Check sheet for the modelled part. Datum: model origin and axes. Units: mm. A direction names the side the tool comes from. Round coordinates to 2 decimals unless told otherwise and drop trailing zeros. Write each loop counter-clockwise with the first axis right and the second up, starting at its lowest first coordinate (ties: lowest second). Pieces come first, ordered by that corner, then holes.
Item 1: Section check B-B, the plane y = 6.5. Record the cut outline in (x, z).
Item 2: Material ranges on line 1 along X through (y, z) = (1.25, 3.5); line 2 along X through (y, z) = (6.25, -0.25); line 3 along Y through (x, z) = (1, 1.5), recorded low to high.
Item 3: Release check for a two-part mould opening along X. For faces 1 (the flat face through (3, 0, 1)), 2 (the flat face through (6.288, 1, 2)), 3 (the flat face through (5, 1, -1.25)) record: pulls with the +X half, pulls with the -X half, needs draft (parallel to the pull), parting line crosses it, or undercut.
Item 4: Section check A-A, the plane z = -2. Record the cut outline in (x, y).
Item 5: Set-up check for faces 4 (the flat face through (3, 1, -1.25)), 5 (the flat face through (3, 1, 3.75)), 6 (the flat face through (-1.182, 1, 3)): record each of +Z, -Z, +X, -X, +Y, -Y from which the full face is reachable in a straight line by a thin tool's end or side.
Item 6: Depth check by flat-ended pin: pin 1 (0.7 mm diameter, centred on y = -0.5, z = -1, fed in from +X); pin 2 (0.8 mm diameter, centred on x = 0, y = 0.5, fed in from -Z); pin 3 (0.5 mm diameter, centred on y = 6, z = 2.5, fed in from -X). Enter the tip coordinate at first touch or a pass-through.
from build123d import *

# Parameters (mm, degrees)
BOSS_EXTRUDE3_DEPTH = 2.54
BOSS_EXTRUDE4_DEPTH = 2.54
LPATTERN1_COUNT     = 2
LPATTERN1_PITCH     = 2.54
BOSS_EXTRUDE5_DEPTH = 0.32
CHAMFER1_SIZE       = 0.16
CHAMFER1_SIZE2      = 0.5458
LPATTERN2_START     = 2.38
LPATTERN2_DEPTH     = 0.32
LPATTERN2_START_2   = 4.92
LPATTERN2_2_DEPTH   = 0.32
LPATTERN2_START_3   = 2.22
LPATTERN2_3_DEPTH   = 0.64
LPATTERN2_START_4   = 4.76
LPATTERN2_4_DEPTH   = 0.64
LPATTERN2_START_5   = -0.32
LPATTERN2_5_DEPTH   = 0.64
LPATTERN2_START_6   = 1
LPATTERN2_6_DEPTH   = 5
SKETCH9_W           = 6.730038924
SKETCH9_H           = 1
BOSS_EXTRUDE6_DEPTH = 2.54


with BuildPart() as part:
    # Sketch6 → Boss-Extrude3 (new body)
    with BuildSketch(Plane(origin=(0, 0, 0), x_dir=(1, 0, 0), z_dir=(0, 1, 0))):
        Polygon((-1.1825, 0.75), (-1.1825, -0.75), (-0.812519462, -1.25), (0.812519462, -1.25), (1.1825, -0.75), (1.1825, 0.75), (0.812519462, 1.25), (-0.812519462, 1.25), align=None)
    extrude(amount=BOSS_EXTRUDE3_DEPTH)

    # Sketch7 → Boss-Extrude4 (add)
    with BuildSketch(Plane(origin=(0, 0, 0), x_dir=(1, 0, 0), z_dir=(0, 1, 0))):
        Polygon((1.1825, 0.75), (1.1825, -0.75), (1.3825, -0.75), (1.752480538, -1.25), (3.377519462, -1.25), (3.7475, -0.75), (3.7475, 0.75), (3.377519462, 1.25), (1.752480538, 1.25), (1.3825, 0.75), align=None)
    boss_extrude4 = extrude(amount=BOSS_EXTRUDE4_DEPTH)

    # LPattern1: Boss-Extrude4 ×2
    with Locations(*[(i * LPATTERN1_PITCH, 0, 0) for i in range(1, LPATTERN1_COUNT)]):
        add(boss_extrude4)

    # Sketch8 → Boss-Extrude5 (add, symmetric)
    with BuildSketch(Plane(origin=(0, 0, 0), x_dir=(0, 0, -1), z_dir=(1, 0, 0))):
        with BuildLine():
            Line((0.32, 0), (0.32, 8))
            Line((0.32, 8), (-0.32, 8))
            Line((-0.32, 8), (-0.32, 0))
            ThreePointArc((-0.32, 0), (-0.13254834, -0.45254834), (0.32, -0.64))
            Line((0.32, -0.64), (2.5, -0.64))
            Line((2.5, -0.64), (2.5, 0))
            Line((2.5, 0), (0.32, 0))
        make_face()
    extrude(amount=BOSS_EXTRUDE5_DEPTH, both=True)

    # Chamfer1
    chamfer1_edges = [part.edges().sort_by_distance(p)[0] for p in [
        (-0.32, 8, 0),
        (0, 8, -0.32),
        (0, 8, 0.32),
        (0.32, 8, 0),
    ]]
    chamfer1_side = [part.faces().sort_by_distance(p)[0] for p in [
        (0, 8, 0),
    ]]
    chamfer(chamfer1_edges, length=CHAMFER1_SIZE, length2=CHAMFER1_SIZE2, reference=chamfer1_side[0])

    # LPattern2: read off the stored shape, not the designer's step
    # LPattern2 outline → LPattern2 (add)
    with BuildSketch(Plane.YZ.offset(LPATTERN2_START)):
        with BuildLine():
            Line((-0.64, -0.32), (-0.64, -2.5))
            Line((-0.64, -2.5), (0, -2.5))
            Line((0, -2.5), (0, 0.32))
            ThreePointArc((0, 0.32), (-0.45254834, 0.13254834), (-0.64, -0.32))
        make_face()
        Polygon((2.54, -0.32), (7.4542, -0.32), (8, -0.16), (8, 0.16), (7.4542, 0.32), (2.54, 0.32), align=None)
    extrude(amount=LPATTERN2_DEPTH)

    # LPattern2 2 outline → LPattern2 2 (add)
    with BuildSketch(Plane.YZ.offset(LPATTERN2_START_2)):
        with BuildLine():
            Line((-0.64, -0.32), (-0.64, -2.5))
            Line((-0.64, -2.5), (0, -2.5))
            Line((0, -2.5), (0, 0.32))
            ThreePointArc((0, 0.32), (-0.45254834, 0.13254834), (-0.64, -0.32))
        make_face()
        Polygon((2.54, -0.32), (7.4542, -0.32), (8, -0.16), (8, 0.16), (7.4542, 0.32), (2.54, 0.32), align=None)
    extrude(amount=LPATTERN2_2_DEPTH)

    # LPattern2 3 outline → LPattern2 3 (add)
    with BuildSketch(Plane.YZ.offset(LPATTERN2_START_3)):
        with BuildLine():
            Line((-0.64, -0.32), (-0.64, -2.5))
            Line((-0.64, -2.5), (0, -2.5))
            Line((0, -2.5), (0, 0.32))
            ThreePointArc((0, 0.32), (-0.45254834, 0.13254834), (-0.64, -0.32))
        make_face()
    extrude(amount=LPATTERN2_3_DEPTH)

    # LPattern2 4 outline → LPattern2 4 (add)
    with BuildSketch(Plane.YZ.offset(LPATTERN2_START_4)):
        with BuildLine():
            Line((-0.64, -0.32), (-0.64, -2.5))
            Line((-0.64, -2.5), (0, -2.5))
            Line((0, -2.5), (0, 0.32))
            ThreePointArc((0, 0.32), (-0.45254834, 0.13254834), (-0.64, -0.32))
        make_face()
    extrude(amount=LPATTERN2_4_DEPTH)

    # LPattern2 5 outline → LPattern2 5 (add)
    with BuildSketch(Plane.XY.offset(LPATTERN2_START_5)):
        Polygon((5.24, 8), (5.24, 2.54), (5.4, 2.54), (5.4, 7.4542), align=None)
        Polygon((4.76, 7.4542), (4.76, 2.54), (4.92, 2.54), (4.92, 8), align=None)
        Polygon((2.7, 8), (2.7, 2.54), (2.86, 2.54), (2.86, 7.4542), align=None)
        Polygon((2.22, 7.4542), (2.22, 2.54), (2.38, 2.54), (2.38, 8), align=None)
    extrude(amount=LPATTERN2_5_DEPTH)

    # LPattern2 6 outline → LPattern2 6 (cut)
    with BuildSketch(Plane.YZ.offset(LPATTERN2_START_6)):
        Polygon((7.4542, 0.32), (8, 0.16), (8, 0.32), align=None)
        Polygon((7.4542, -0.32), (8, -0.32), (8, -0.16), align=None)
    extrude(amount=LPATTERN2_6_DEPTH, mode=Mode.SUBTRACT)

    # Mirror1: part across plane


with BuildPart() as part_1:
    add(part.part)
    add(part.part.mirror(Plane(origin=(-0.812519462, 2.54, 1.25), x_dir=(1, 0, 0), z_dir=(0, 0, -1))))

    # Sketch9 → Boss-Extrude6 (add)
    with BuildSketch(Plane.XZ):
        with Locations((2.5525, 1.25)):
            Rectangle(SKETCH9_W, SKETCH9_H)
    extrude(amount=-BOSS_EXTRUDE6_DEPTH)


solid = part_1.part
Values found:
1. outline: (-0.32, -0.32) - (0.32, -0.32) - (0.32, 0.32) - (-0.32, 0.32) - close; (-0.32, 2.18) - (0.32, 2.18) - (0.32, 2.82) - (-0.32, 2.82) - close; (2.22, -0.32) - (2.86, -0.32) - (2.86, 0.32) - (2.22, 0.32) - close; (2.22, 2.18) - (2.86, 2.18) - (2.86, 2.82) - (2.22, 2.82) - close; (4.76, -0.32) - (5.4, -0.32) - (5.4, 0.32) - (4.76, 0.32) - close; (4.76, 2.18) - (5.4, 2.18) - (5.4, 2.82) - (4.76, 2.82) - close
2. line 1: x = -1 to 1, 1.57 to 3.56, 4.11 to 6.1
2. line 2: x = -0.32 to 0.32, 2.22 to 2.86, 4.76 to 5.4
2. line 3: y = 0 to 2.54
3. face 1: undercut
3. face 2: pulls with the +X half
3. face 3: needs draft
4. outline: (-0.32, -0.64) - (0.32, -0.64) - (0.32, 0) - (-0.32, 0) - close; (2.22, -0.64) - (2.86, -0.64) - (2.86, 0) - (2.22, 0) - close; (4.76, -0.64) - (5.4, -0.64) - (5.4, 0) - (4.76, 0) - close
5. face 4: -Z, +X, -X, +Y
5. face 5: +Z, +X, -X, +Y
5. face 6: +Z, -Z, -X, +Y, -Y
6. pin 1: stops at x = 5.4
6. pin 2: stops at z = -1.25
6. pin 3: stops at x = -0.32
